from build123d import *

# Parameters (mm, degrees)
SKETCH1_R           = 1.7
BOSS_EXTRUDE1_DEPTH = 3.175


with BuildPart() as part:
    # Sketch1 → Boss-Extrude1 (new body)
    with BuildSketch(Plane(origin=(0, 0, 0), x_dir=(-1, 0, 0), z_dir=(0, 0, -1))):
        with BuildLine():
            Line((5.417282063, -59.58290593), (5.417282063, 171.394622999))
            ThreePointArc((5.417282063, 171.394622999), (-24.582717937, 201.394622999), (-54.582717937, 171.394622999))
            Line((-54.582717937, 171.394622999), (-54.582717937, -59.58290593))
            ThreePointArc((-54.582717937, -59.58290593), (-24.582717937, -89.58290593), (5.417282063, -59.58290593))
        make_face()
        with Locations((2.167282063, 52.505858535)):
            Circle(SKETCH1_R, mode=Mode.SUBTRACT)
        with Locations((-51.332717937, 59.305858535)):
            Circle(SKETCH1_R, mode=Mode.SUBTRACT)
        with Locations((-51.332717937, 52.505858535)):
            Circle(SKETCH1_R, mode=Mode.SUBTRACT)
        with Locations((-21.282717937, 197.940291196)):
            Circle(SKETCH1_R, mode=Mode.SUBTRACT)
        with Locations((2.167282063, -4.094141465)):
            Circle(SKETCH1_R, mode=Mode.SUBTRACT)
        with Locations((-51.332717937, -4.094141465)):
            Circle(SKETCH1_R, mode=Mode.SUBTRACT)
        with Locations((-51.332717937, -59.58290593)):
            Circle(SKETCH1_R, mode=Mode.SUBTRACT)
        with Locations((2.167282063, 115.905858535)):
            Circle(SKETCH1_R, mode=Mode.SUBTRACT)
        with Locations((-51.332717937, 115.905858535)):
            Circle(SKETCH1_R, mode=Mode.SUBTRACT)
        with Locations((2.167282063, 171.394622999)):
            Circle(SKETCH1_R, mode=Mode.SUBTRACT)
        with Locations((-27.982717937, -86.115951364)):
            Circle(SKETCH1_R, mode=Mode.SUBTRACT)
        with Locations((2.167282063, 59.305858535)):
            Circle(SKETCH1_R, mode=Mode.SUBTRACT)
        with Locations((-51.332717937, 171.394622999)):
            Circle(SKETCH1_R, mode=Mode.SUBTRACT)
        with Locations((-21.182717937, -86.115951364)):
            Circle(SKETCH1_R, mode=Mode.SUBTRACT)
        with Locations((2.167282063, -59.58290593)):
            Circle(SKETCH1_R, mode=Mode.SUBTRACT)
        with Locations((-27.882717937, 197.940291196)):
            Circle(SKETCH1_R, mode=Mode.SUBTRACT)
    extrude(amount=-BOSS_EXTRUDE1_DEPTH)


solid = part.part
Design review of the part built by this model. Coordinates are the model's own, in mm. Round coordinates to 2 decimals unless told otherwise and drop trailing zeros. Order: outer loops, then holes, each group sorted by start corner. A loop starts at its lowest first (then second) coordinate and runs counter-clockwise, first axis right, second up.
1) Clearance check with a flat-ended pin moving along its axis: pin 1 Ø2 at (x, y) = (-2.17, 115.91) entering from +Z. State where the tip first meets the part, or that it passes through.
The answers:
pin 1: passes through
2) For L1, parallel to X at y = 114.5, z = 0.55; L2, parallel to X at y = 170.5, z = 3.05; L3, parallel to Y at x = 14, z = 2, list the stretches that pass through material, from the lowest coordinate up.
The answers:
L1: x = -5.42 to -3.12, -1.21 to 50.38, 52.29 to 54.58
L2: x = -5.42 to -3.61, -0.72 to 49.89, 52.78 to 54.58
L3: y = -87.65 to 199.47
3) Consider section C-C (x = 8). State the section outline as (y, z) points (3 decimals).
The answers:
outline: (-84.583, 0) - (196.395, 0) - (196.395, 3.175) - (-84.583, 3.175) - close
4) Consider section A-A (z = 1.8). Count the separate pieces of the cut face and the enclosed holes in it, plus the area to 3 significant figures.
The answers:
separate pieces: 1
enclosed holes: 16
area: 16,500 mm2
5) Consider section B-B (x = 37). State the section outline as (y, z) points (3 decimals), plus the area to 3 significant figures.
The answers:
outline: (-86.892, 0) - (198.704, 0) - (198.704, 3.175) - (-86.892, 3.175) - close
area: 907 mm2
